```python
from build123d import *

# Parameters (mm, degrees)
SKETCH1_R            = 6
BOSS_EXTRUDE1_DEPTH  = 6.35
M5_CLEARANCE_HOLE1_D = 5.3


with BuildPart() as part:
    # Sketch1 → Boss-Extrude1 (new body)
    with BuildSketch(Plane(origin=(0, 0, 0), x_dir=(1, 0, 0), z_dir=(0, 1, 0))):
        with BuildLine():
            Line((-20, 0), (-14.99481954, -190.394191531))
            ThreePointArc((-14.99481954, -190.394191531), (0, -205), (14.99481954, -190.394191531))
            Line((14.99481954, -190.394191531), (20, 0))
            ThreePointArc((20, 0), (0, 20), (-20, 0))
        make_face()
        with Locations((0, -190)):
            Circle(SKETCH1_R, mode=Mode.SUBTRACT)
    extrude(amount=BOSS_EXTRUDE1_DEPTH)

    # M5 Clearance Hole1 (through all)
    with Locations(Plane(origin=(0, 6.35, 0), x_dir=(1, 0, 0), z_dir=(0, 1, 0))):
        with Locations((-10, 0), (10, 0)):
            Hole(M5_CLEARANCE_HOLE1_D / 2)


solid = part.part
```
Work out the finished part from the listing and answer in its coordinate system (mm). Round coordinates to 2 decimals unless told otherwise and drop trailing zeros. Loops run counter-clockwise (first coordinate to the right, second up) from the corner with the lowest first, then second, coordinate; pieces in that order, holes last. Notation, with made-up numbers: M -19.5,3.5 L -2.5,3.5 A26 cw -2.5,20.5 Z; hole C 65,31.5 d5. An arc over 180 degrees is marked long. Use CSV: the item, a comma, the result in double quotes.
Q1. Section C-C, the plane x = 10 is taken. Determine the outline of the cut face in (y, z), then the cut area to 3 significant figures.
Determined:
outline,"M 0,-17.32 L 6.35,-17.32 L 6.35,-2.65 L 0,-2.65 Z; M 0,2.65 L 6.35,2.65 L 6.35,201.18 L 0,201.18 Z"
area,"1,350 mm2"
Q2. Consider L1, parallel to Z at x = 0, y = 5.25; L2, parallel to Z at x = -1.5, y = 3.5; L3, parallel to X at y = 1, z = 136. Determine where each line is inside the solid, lowest interval first.
Determined:
L1,"-20 to 184, 196 to 205"
L2,"-19.94 to 184.19, 195.81 to 204.92"
L3,"-16.42 to 16.42"
Q3. Section A-A, the plane y = 4 is taken. Determine the outline of the cut face in (x, z), then the cut area to 3 significant figures.
Determined:
outline,"M -20,0 A20 ccw 20,0 L 14.99,190.39 A15 ccw -14.99,190.39 Z; hole C -10,0 d5.3; hole C 0,190 d12; hole C 10,0 d5.3"
area,"7,480 mm2"
Q4. The mould has two halves that part along X. Classify faces 1 (the cylindrical face through (12.647, 3.131, -0.117)), 2 (the cylindrical face through (0, 3, -20)), 3 (the flat face through (0, 0, 91)): pulls with the +X half, pulls with the -X half, needs draft (parallel to the pull), parting line crosses it, or undercut.
Determined:
face 1,"undercut"
face 2,"parting line crosses it"
face 3,"needs draft"
Q5. Section B-B, the plane x = 0 is taken. Determine the outline of the cut face in (y, z), then the cut area to 3 significant figures.
Determined:
outline,"M 0,-20 L 6.35,-20 L 6.35,184 L 0,184 Z; M 0,196 L 6.35,196 L 6.35,205 L 0,205 Z"
area,"1,350 mm2"
Q6. Each of these flat-tipped pins is pushed along its axis until it touches: pin 1 (4 mm diameter, centred on x = -10, z = 0, fed in from +Y); pin 2 (1.5 mm diameter, centred on x = -4, y = 5.5, fed in from +Z); pin 3 (3 mm diameter, centred on y = 5.5, z = 77.5, fed in from +X); pin 4 (3 mm diameter, centred on y = 2, z = 98, fed in from +X). Where does it stop, or does it pass through?
Determined:
pin 1,"through"
pin 2,"z = 204.64"
pin 3,"x = 18"
pin 4,"x = 17.46"
Q7. Section D-D, the plane z = 18 is taken. Determine the outline of the cut face in (x, y).
Determined:
outline,"M -19.53,0 L 19.53,0 L 19.53,6.35 L -19.53,6.35 Z"
